Source: CAD feature listing. Evaluate the final solid. Frame: model axes, mm. Coordinates: 2 decimals unless noted, no trailing zeros. Write each loop counter-clockwise with the first axis right and the second up, starting at its lowest first coordinate (ties: lowest second). Pieces come first, ordered by that corner, then holes. Notation, with made-up numbers: (77, -6) - (88, -6) arc R17 cw to (88, 19) - close; hole circle Ø7 at (1.25, 88.5). An arc over 180 degrees is marked (long way). One line per item, written item: value.
from build123d import *

# Parameters (mm, degrees)
BOSS_EXTRUDE1_DEPTH = 4


with BuildPart() as part:
    # Sketch1 → Boss-Extrude1 (new body)
    with BuildSketch(Plane.XY):
        with BuildLine():
            ThreePointArc((3.396226415, -2.113207547), (0, -4), (-3.396226415, -2.113207547))
            Line((-3.396226415, -2.113207547), (0, -14))
            Line((0, -14), (3.396226415, -2.113207547))
        make_face()
        with BuildLine():
            Line((-2, 0), (-4, 0))
            Line((-4, 0), (-3.396226415, -2.113207547))
            ThreePointArc((-3.396226415, -2.113207547), (0, -4), (3.396226415, -2.113207547))
            Line((3.396226415, -2.113207547), (4, 0))
            Line((4, 0), (2, 0))
            ThreePointArc((2, 0), (0, -2), (-2, 0))
        make_face()
        with BuildLine():
            ThreePointArc((4, 0), (0, 4), (-4, 0))
            Line((-4, 0), (-2, 0))
            ThreePointArc((-2, 0), (0, 2), (2, 0))
            Line((2, 0), (4, 0))
        make_face()
    extrude(amount=BOSS_EXTRUDE1_DEPTH)


solid = part.part
1) Material intervals for line 1 (X direction, y = 0.25, z = 0.5); line 2 (X direction, y = 2.5, z = 2.65); line 3 (X direction, y = -1.75, z = 1.05), sorted ascending.
Values found:
line 1: -3.99 to -1.98, 1.98 to 3.99
line 2: -3.12 to 3.12
line 3: -3.5 to -0.97, 0.97 to 3.5
2) Section query D-D on y = -8. Output: boundary loops of the cut face in (x, z).
Values found:
outline: (-1.71, 0) - (1.71, 0) - (1.71, 4) - (-1.71, 4) - close
3) Section query C-C on x = -1. Output: boundary loops of the cut face in (y, z), then the cut area to 3 significant figures.
Values found:
outline: (-10.5, 0) - (-1.73, 0) - (-1.73, 4) - (-10.5, 4) - close; (1.73, 0) - (3.87, 0) - (3.87, 4) - (1.73, 4) - close
area: 43.6 mm2
4) Section query B-B on z = 0.55. Output: boundary loops of the cut face in (x, y).
Values found:
outline: (-4, 0) - (0, -14) - (4, 0) arc R4 ccw to start; hole circle Ø4 at (0, 0)
5) Section query A-A on y = -1.75. Output: boundary loops of the cut face in (x, z).
Values found:
outline: (-3.5, 0) - (-0.97, 0) - (-0.97, 4) - (-3.5, 4) - close; (0.97, 0) - (3.5, 0) - (3.5, 4) - (0.97, 4) - close
6) Contact query for flat-ended pins moving along their axis: P1, Ø1.5, axis at y = -5.5, z = 1, coming from the -X side; P2, Ø1.5, axis at y = -11.5, z = 0.5, coming from the +X side; P3, Ø2, axis at y = -4.5, z = 1, coming from the -X side. Output: stop coordinate, or through.
Values found:
P1: x = -2.64
P2: x = 0.93
P3: x = -3
7) Draft query along Y for faces 1 (the flat face through (0, -3, 0)), 2 (the cylindrical face through (0, -2, 2)), 3 (the cylindrical face through (0, 4, 2)). Return one class per face: released by +Y, released by -Y, zero draft, split by the parting line, or undercut.
Values found:
face 1: zero draft
face 2: undercut
face 3: released by +Y
